Could you check a few things on this model? Use its own coordinates, in mm. Face numbers are marked on the shaded views. Round coordinates to 2 decimals unless told otherwise and drop trailing zeros. Loops run counter-clockwise (first coordinate to the right, second up) from the corner with the lowest first, then second, coordinate; pieces in that order, holes last. Notation, with made-up numbers: M 28,54.25 L 87,54.25 A24 cw 87,70.25 Z; hole C 55,51.25 d6. An arc over 180 degrees is marked long. One line per item, written item: value. Start each with the question number.
Q1. Thinking about a two-plate mould opening in Y: for the marked faces 1, 2 and 3, which applies, released by +Y, released by -Y, zero draft, split by the parting line, or undercut?
Q2. Please list where these lines run through material, in increasing order: line 1 along Z through (x, y) = (3.25, 16); line 2 along Z through (x, y) = (6, -23.5); line 3 along Z through (x, y) = (-1, -33).
Q3. Imagine slicing it at D-D (y = 14). Please give me the cut outline in (x, z).
Q4. I'm going to push flat-ended pins straight in: pin 1 Ø4 at (y, z) = (-25.5, -3) entering from +X; pin 2 Ø1.5 at (y, z) = (7, 3.5) entering from +X; pin 3 Ø4 at (y, z) = (-28.5, -9) entering from +X. Where does each tip first touch, or does it pass through?
Q5. Imagine slicing it at C-C (y = -16.5). Please give me the cut outline in (x, z).
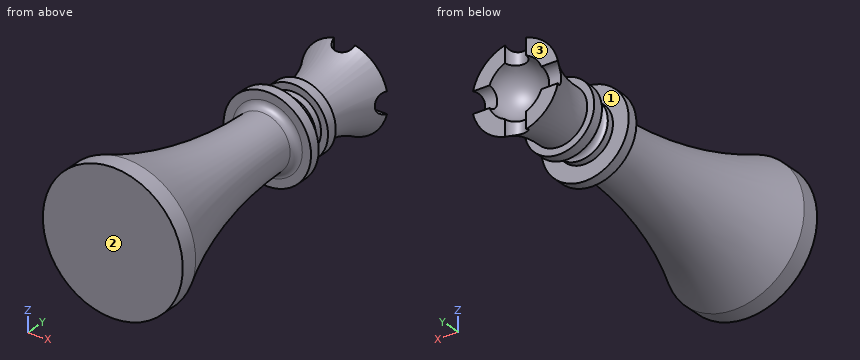
from build123d import *

# Parameters (mm, degrees)
CUT_EXTRUDE1_REACH            = 68.332
CUT_EXTRUDE1_END_MAJOR_RADIUS = 37.977551241
CUT_EXTRUDE1_END_MINOR_RADIUS = 30
SKETCH2_R                     = 3
CIRPATTERN1_COUNT             = 4
SCALE_1_SCALE                 = 0.6


with BuildPart() as part:
    # Sketch1 → Revolve1 (revolve)
    with BuildSketch(Plane.XY, mode=Mode.PRIVATE) as revolve1_sk:
        with BuildLine():
            Line((0, -60), (20, -60))
            Line((20, -60), (20, -55))
            ThreePointArc((20, -55), (11.206794692, -29.145390653), (8.008821921, -2.024287169))
            ThreePointArc((8.008821921, -2.024287169), (8.585899987, -0.594399477), (10.008674448, 0))
            Line((10.008674448, 0), (12.5, 0))
            Line((12.5, 0), (12.5, 3))
            Line((12.5, 3), (8, 3))
            Line((8, 3), (8, 5))
            ThreePointArc((8, 5), (6.5, 6.5), (8, 8))
            Line((8, 8), (8, 10))
            Line((8, 10), (10, 10))
            Line((10, 10), (10, 13))
            Line((10, 13), (8, 13))
            ThreePointArc((8, 13), (8.976394405, 21.837130893), (12.5, 30))
            Line((12.5, 30), (8, 30))
            ThreePointArc((8, 30), (5.656854249, 24.343145751), (0, 22))
            Line((0, 22), (0, -60))
        make_face()
    revolve(revolve1_sk.sketch.rotate(Axis((0, 0, 0), (0, 1, 0)), 90), axis=Axis((0, 0, 0), (0, 1, 0)))

    # Cut-Extrude1: up to this torus (the profile starts outside it)
    cut_extrude1_end = Plane(origin=(0, 14.160354083, 0), z_dir=(0, -1, 0)) * Torus(CUT_EXTRUDE1_END_MAJOR_RADIUS, CUT_EXTRUDE1_END_MINOR_RADIUS, mode=Mode.PRIVATE)
    # Sketch2 → Cut-Extrude1 (cut, up to the surface)
    with BuildSketch(Plane.XY, mode=Mode.PRIVATE) as cut_extrude1_sk1:
        with Locations((0, 30)):
            Circle(SKETCH2_R)
    cut_extrude1_tool1 = extrude(cut_extrude1_sk1.sketch, amount=-CUT_EXTRUDE1_REACH, mode=Mode.PRIVATE) - cut_extrude1_end
    cut_extrude1 = cut_extrude1_tool1.solids().sort_by_distance((0, 30, 0))[0]
    add(cut_extrude1, mode=Mode.SUBTRACT)

    # CirPattern1: Cut-Extrude1 ×4 about axis
    cirpattern1_axis = Axis((0, 13, 0), (0, -1, 0))
    for i in range(1, CIRPATTERN1_COUNT):
        add(cut_extrude1.rotate(cirpattern1_axis, i * 360 / CIRPATTERN1_COUNT), mode=Mode.SUBTRACT)


with BuildPart() as part_1:
    # 缩放比例1: scaled about (0, 0, 0)
    add(part.part.scale(SCALE_1_SCALE))


solid = part_1.part
Report:
1. face 1: undercut
1. face 2: released by -Y
1. face 3: released by +Y
2. line 1: z = -5.54 to -2.91, 2.91 to 5.54
2. line 2: z = -5.79 to 5.79
2. line 3: z = -11.96 to 11.96
3. outline: C 0,0 d11.3; hole C 0,0 d5.31
4. pin 1: stops at x = 9.4
4. pin 2: stops at x = 5.33
4. pin 3: stops at x = 7.56
5. outline: C 0,0 d13.01
